CAD build for the part. Positions are in the model's coordinates, mm. A direction names the side the tool comes from. Give positions to 0.01 mm unless a question says otherwise; leave off trailing zeros. Write each loop counter-clockwise with the first axis right and the second up, starting at its lowest first coordinate (ties: lowest second). Pieces come first, ordered by that corner, then holes. Notation, with made-up numbers: M -12.75,60 L 17.25,60 A12 ccw 17.25,74 Z; hole C 48,14 d1. An arc over 180 degrees is marked long. One line per question, with ' | ' between items. Start each with the question number.
1. Wall check: L1, parallel to X at y = 14.5, z = -4.75; L2, parallel to Z at x = 2.5, y = 17; L3, parallel to Y at x = 7.5, z = -0.5. Give the ranges that are in metal, low to high.
2. Cut at C-C, the plane y = 3.5. Write the cut outline in (x, z), then the cut area to 3 significant figures.
3. Cut at A-A, the plane z = 0. Write the cut outline in (x, y), then the cut area to 3 significant figures.
4. Flat gauge pins, fed straight in: pin 1 (6 mm diameter, centred on y = 20.5, z = -6, fed in from -X); pin 2 (1.5 mm diameter, centred on x = -2.5, y = 27, fed in from +Z); pin 3 (6 mm diameter, centred on x = 1, z = -6.5, fed in from +Y). Where does each tip first touch, or does it go through?
5. Which spindle directions (+Z, -Z, +X, -X, +Y, -Y) get a long thin tool onto all of the face, cutting with end or side? Do faces 1 (the face through (0, 0, 0)), 2 (the face through (-0.867, 5.916, 3.905)). Say none if no direction does.
6. Cut at D-D, the plane z = -3.5. Write the cut outline in (x, y).
7. Pull direction X, two halves, no side cores. Call faces 3 (the face through (-1.172, 15.451, -8.923)), 4 (the face through (4, 12, 2)): released by +X, released by -X, zero draft, split by the parting line, or undercut.
8. Cut at B-B, the plane x = 0. Write the cut outline in (y, z), then the cut area to 3 significant figures.
```python
from build123d import *

# Parameters (mm, degrees)
SKETCH1_R           = 4
BOSS_EXTRUDE1_DEPTH = 12
SKETCH3_R           = 9
BOSS_EXTRUDE2_DEPTH = 7


with BuildPart() as part:
    # Sketch1 → Boss-Extrude1 (new body)
    with BuildSketch(Plane(origin=(0, 0, 0), x_dir=(1, 0, 0), z_dir=(0, 1, 0))):
        Circle(SKETCH1_R)
    extrude(amount=BOSS_EXTRUDE1_DEPTH)

    # Sketch3 → Boss-Extrude2 (add)
    with BuildSketch(Plane(origin=(0, 12, 0), x_dir=(1, 0, 0), z_dir=(0, 1, 0))):
        Circle(SKETCH3_R)
    extrude(amount=BOSS_EXTRUDE2_DEPTH)

    # Sketch4 → Revolve2 (revolve)
    with BuildSketch(Plane.XY):
        with BuildLine():
            Line((0, 28.11938617), (0, 19))
            Line((0, 19), (9, 19))
            ThreePointArc((9, 19), (8.596342111, 28.841142067), (0, 33.648835815))
            Line((0, 33.648835815), (0, 28.11938617))
        make_face()
    revolve(axis=Axis((0, 28.11938617, 0), (0, -1, 0)))


solid = part.part
```
Here are the results:
1) L1: -7.64 to 7.64 | L2: -8.65 to 8.65 | L3: 12 to 30.29
2) outline: C 0,0 d8 | area: 50.3 mm^2
3) outline: M -9,12 L -4,12 L -4,0 L 4,0 L 4,12 L 9,12 L 9,19 A10.09 ccw long -9,19 Z | area: 471 mm^2
4) pin 1: x = -9.37 | pin 2: z = 9.46 | pin 3: y = 32.99
5) face 1: +Z, -Z, +X, -X, -Y | face 2: -Y
6) outline: M -8.29,12 L -1.94,12 L -1.94,0 L 1.94,0 L 1.94,12 L 8.29,12 L 8.29,19 A9.46 ccw long -8.29,19 Z
7) face 3: split by the parting line | face 4: zero draft
8) outline: M 0,-4 L 12,-4 L 12,-9 L 19,-9 A10.09 ccw long 19,9 L 12,9 L 12,4 L 0,4 Z | area: 471 mm^2
